```python
from build123d import *


with BuildPart() as f1:
    # F0 (on Front) → F1 (revolve)
    with BuildSketch(Plane.XZ):
        Polygon((8, 49.8), (3, 49.8), (2.555618, 49.211922), (2.555618, 48.211922), (3.687895, 45.965945), (3.687895, 41.892459), (2.2, 39.236551), (2.2, 7.1), (2.2, 0), (2.476728, 0), (3.047144, 0.404497), (3.047144, 4.667719), (2.476728, 5), (2.476728, 7.1), (11.011527, 7.1), (11.011527, 8.032141), (3, 8.032141), (3, 10.032141), (11.011527, 10.032141), (11.011527, 11.032141), (3, 11.032141), (3, 13.232141), (11.011527, 13.232141), (11.011527, 14.232141), (3, 14.232141), (3, 16.432141), (11.011527, 16.432141), (11.011527, 17.432141), (3, 17.432141), (3, 19.532141), (11, 19.532141), (11, 20.532141), (6.5, 20.532141), (6.5, 21.932141), (11, 21.932141), (11, 22.932141), (3, 22.932141), (3, 25.032141), (11, 25.032141), (11, 26.032141), (3, 26.032141), (3, 29.032141), (11, 29.032141), (11, 30.032141), (3, 30.032141), (3, 32.132141), (11, 32.132141), (11, 33.132141), (4.5, 33.132141), (4.5, 34.524906), (8, 34.524906), (8, 35.524906), (4.5, 35.524906), (4.5, 37.1), (8, 37.1), (8, 40.1), (6, 40.1), (6, 46.1), (8, 46.1), align=None)
    revolve(axis=Axis((0, 0, 18.136091), (0, 0, -1)))


solid = f1.part
```
Verification items for the finished model (mm, model axes). A direction names the side the tool comes from. Give positions to 0.01 mm unless a question says otherwise; leave off trailing zeros. Loops run counter-clockwise (first coordinate to the right, second up) from the corner with the lowest first, then second, coordinate; pieces in that order, holes last. Notation, with made-up numbers: M 7.25,71 L 34.25,71 A23 ccw 34.25,91 Z; hole C 44.5,58 d5. An arc over 180 degrees is marked long. Return JSON: item names as keys, results as strings.
1) Tool access check on faces 4 (the cylindrical face through (-0.4, -3.02, 2.57)), 5 (the cylindrical face through (-1.73, 7.81, 35.03)), 6 (the flat face through (-2.3, 2.3, 10.032)). Record the directions out of +Z, -Z, +X, -X, +Y, -Y that give a thin tool (end or side, any length) a straight path to the whole face; none if there is none.
Findings:
{"face 4": "-Z", "face 5": "+Z", "face 6": "none"}
2) Section check A-A, the plane z = 24.5. Enter the section's corners in (x, y).
Findings:
{"outline": "C 0,0 d6; hole C 0,0 d4.4"}
3) Material ranges on L1, parallel to X at y = 0, z = 13; L2, parallel to X at y = 0, z = 21, recorded low to high. Write a range as [from, to].
Findings:
{"L1": "x = [-3, -2.2], [2.2, 3]", "L2": "x = [-6.5, -2.2], [2.2, 6.5]"}
4) Section check B-B, the plane y = -7.5. Count the separate pieces of the cut face and the enclosed holes in it, and give its area (3 significant figures).
Findings:
{"separate pieces": "12", "enclosed holes": "0", "area": "187 mm2"}
5) Mould release check, pull along X, two halves, no side actions. Record for faces 1 (the cylindrical face through (2.1, -0.66, 19.34)), 2 (the cylindrical face through (-3, 0, 28)), 3 (the flat face through (3, 0, 7.1)): released by +X, released by -X, zero draft, split by the parting line, or undercut.
Findings:
{"face 1": "undercut", "face 2": "split by the parting line", "face 3": "zero draft"}
6) Gauge pin test, flat ends, axial feed: P1, Ø2, axis at x = 0, y = 0, coming from the -Z side; P2, Ø12, axis at x = -8, y = 6, coming from the -Z side; P3, Ø3, axis at x = -2.5, z = 28.5, coming from the +Y side; P4, Ø11, axis at x = -3.5, y = -3, coming from the -Z side. Record the tip position at first contact, or that the pin passes through.
Findings:
{"P1": "passes through", "P2": "stops at z = 7.1", "P3": "stops at y = 10.95", "P4": "stops at z = 0"}
